The figure shows three views and two pictorial views of one solid part (mm, origin at its lowest corner). Answer the questions. Give positions to 0.01 mm unless a question says otherwise; leave off trailing zeros. Order: outer loops, then holes, each group sorted by start corner. A loop starts at its lowest first (then second) coordinate and runs counter-clockwise, first axis right, second up. Notation, with made-up numbers: (8.5, 20) - (39.5, 20) arc R27 ccw to (39.5, 52) - close; hole circle Ø9 at (10, 15). An arc over 180 degrees is marked (long way). Return JSON: item names as keys, results as strings. Group by question number.
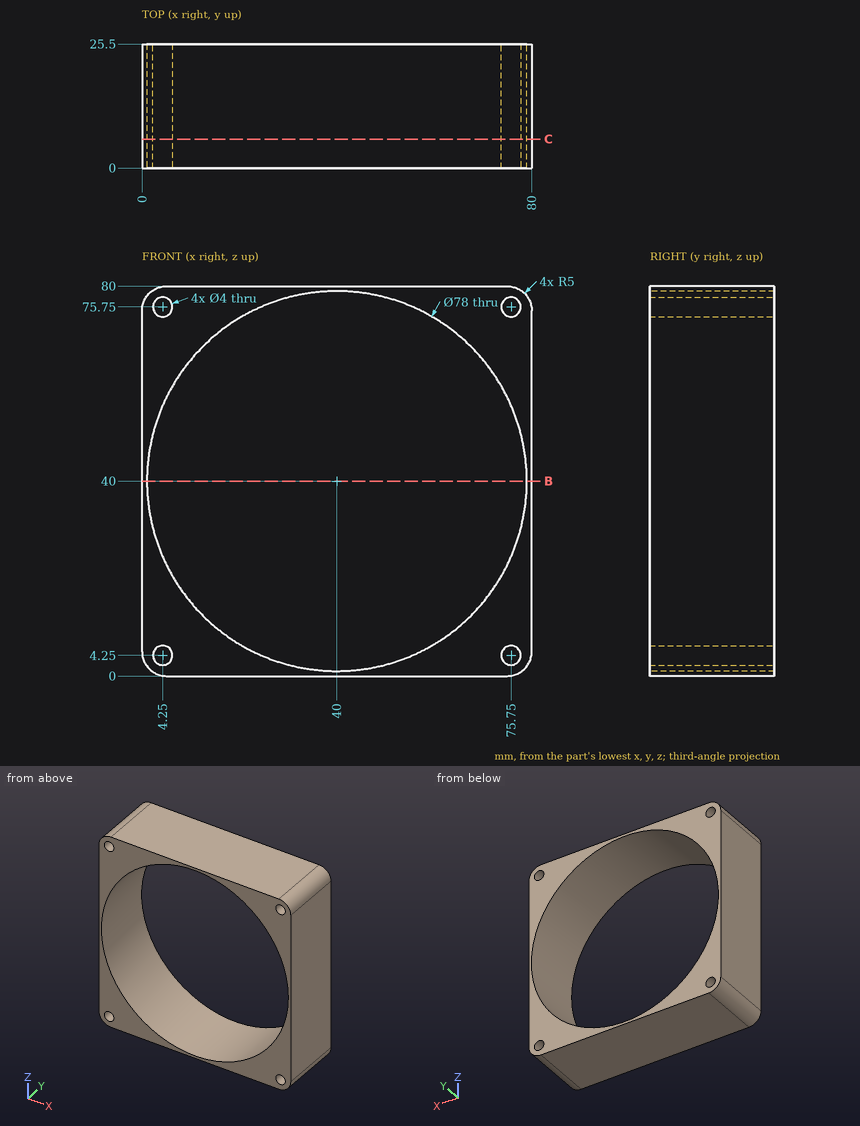
1. The part is cut by section C-C (y = 6). Give the vertices of the cut face in (x, z), and give its area (3 significant figures).
2. Consider probe 1 along Z at (x, y) = (4.25, 10.5); probe 2 along Z at (x, y) = (39.5, 23.5); probe 3 along X at (y, z) = (3.5, 61.5). Determine where each line is inside the solid, lowest interval first. Write a range as from..to.
3. The part is cut by section B-B (z = 40). Give the vertices of the cut face in (x, y), and give its area (3 significant figures).
4. This flat-tipped pin is pushed along its axis until it touches: pin 1 (3.5 mm diameter, centred on x = 75.75, z = 75.75, fed in from -Y). Where does it stop, or does it pass through?
Answers:
{
 "1": {"outline": "(0, 5) arc R5 ccw to (5, 0) - (75, 0) arc R5 ccw to (80, 5) - (80, 75) arc R5 ccw to (75, 80) - (5, 80) arc R5 ccw to (0, 75) - close; hole circle Ø78 at (40, 40); hole circle Ø4 at (4.25, 4.25); hole circle Ø4 at (4.25, 75.75); hole circle Ø4 at (75.75, 4.25); hole circle Ø4 at (75.75, 75.75)", "area": "1,550 mm^2"},
 "2": {"probe 1": "z = 0.06..2.25, 6.25..24.41, 55.59..73.75, 77.75..79.94", "probe 2": "z = 0..1, 79..80", "probe 3": "x = 0..7.46, 72.54..80"},
 "3": {"outline": "(0, 0) - (1, 0) - (1, 25.5) - (0, 25.5) - close; (79, 0) - (80, 0) - (80, 25.5) - (79, 25.5) - close", "area": "51.0 mm^2"},
 "4": {"pin 1": "passes through"}
}
